from build123d import *

# Parameters (mm, degrees)
SKETCH1_R           = 2.0701
SKETCH1_R_2         = 2.4892
BOSS_EXTRUDE1_DEPTH = 2.54


with BuildPart() as part:
    # Sketch1 → Boss-Extrude1 (new body)
    with BuildSketch(Plane.XY):
        with BuildLine():
            Line((-35.539454624, 50.8), (60.96, 50.8))
            ThreePointArc((60.96, 50.8), (62.756051224, 50.056051224), (63.5, 48.26))
            Line((63.5, 48.26), (63.5, 27.94))
            ThreePointArc((63.5, 27.94), (62.756051224, 26.143948776), (60.96, 25.4))
            Line((60.96, 25.4), (39.37, 25.4))
            ThreePointArc((39.37, 25.4), (33.981846327, 23.168153673), (31.75, 17.78))
            Line((31.75, 17.78), (31.75, -3.81))
            ThreePointArc((31.75, -3.81), (31.006051224, -5.606051224), (29.21, -6.35))
            Line((29.21, -6.35), (-3.81, -6.35))
            ThreePointArc((-3.81, -6.35), (-5.606051224, -5.606051224), (-6.35, -3.81))
            Line((-6.35, -3.81), (-6.35, 17.78))
            ThreePointArc((-6.35, 17.78), (-8.581846327, 23.168153673), (-13.97, 25.4))
            Line((-13.97, 25.4), (-35.539454624, 25.4))
            ThreePointArc((-35.539454624, 25.4), (-37.335505848, 26.143948776), (-38.079454624, 27.94))
            Line((-38.079454624, 27.94), (-38.079454624, 48.26))
            ThreePointArc((-38.079454624, 48.26), (-37.335505848, 50.056051224), (-35.539454624, 50.8))
        make_face()
        with Locations((-25.4, 38.1)):
            Circle(SKETCH1_R, mode=Mode.SUBTRACT)
        with Locations((0, 38.1)):
            Circle(SKETCH1_R, mode=Mode.SUBTRACT)
        with Locations((25.4, 38.1)):
            Circle(SKETCH1_R, mode=Mode.SUBTRACT)
        with Locations((50.8, 38.1)):
            Circle(SKETCH1_R, mode=Mode.SUBTRACT)
        with Locations((0, 12.7)):
            Circle(SKETCH1_R_2, mode=Mode.SUBTRACT)
        Circle(SKETCH1_R_2, mode=Mode.SUBTRACT)
        with Locations((25.4, 12.7)):
            Circle(SKETCH1_R_2, mode=Mode.SUBTRACT)
        with Locations((25.4, 0)):
            Circle(SKETCH1_R_2, mode=Mode.SUBTRACT)
    extrude(amount=BOSS_EXTRUDE1_DEPTH)


solid = part.part
Input: part model. Units: mm. Frame: model coordinates. A direction names the side the tool comes from. Give positions to 0.01 mm unless a question says otherwise; leave off trailing zeros. Write each loop counter-clockwise with the first axis right and the second up, starting at its lowest first coordinate (ties: lowest second). Pieces come first, ordered by that corner, then holes. Notation, with made-up numbers: M 17,55 L 24,55 A13 cw 24,76 Z; hole C 77.5,78 d6. An arc over 180 degrees is marked long. Use one line per item in the form item = value.
1. Ray query, L1, parallel to Y at x = 0, z = 1.45; L2, parallel to X at y = 38.5, z = 0.5; L3, parallel to Y at x = -25.5, z = 0.3. Return the intervals inside material, ascending.
Outcome:
L1 = -6.35 to -2.49, 2.49 to 10.21, 15.19 to 36.03, 40.17 to 50.8
L2 = -38.08 to -27.43, -23.37 to -2.03, 2.03 to 23.37, 27.43 to 48.77, 52.83 to 63.5
L3 = 25.4 to 36.03, 40.17 to 50.8
2. Cut plane B-B on y = 38.1. Return loops of the section in (x, z), and give its area (3 significant figures).
Outcome:
outline = M -38.08,0 L -27.47,0 L -27.47,2.54 L -38.08,2.54 Z; M -23.33,0 L -2.07,0 L -2.07,2.54 L -23.33,2.54 Z; M 2.07,0 L 23.33,0 L 23.33,2.54 L 2.07,2.54 Z; M 27.47,0 L 48.73,0 L 48.73,2.54 L 27.47,2.54 Z; M 52.87,0 L 63.5,0 L 63.5,2.54 L 52.87,2.54 Z
area = 216 mm²
3. Cut plane D-D on z = 1.05. State how many separate pieces and enclosed holes the cut face has, and give its area (3 significant figures).
Outcome:
separate_pieces = 1
enclosed_holes = 8
area = 3,670 mm²
4. First-contact query: P1, Ø1.3, axis at x = 48, z = 1, coming from the -Y side; P2, Ø2.5, axis at x = 25.4, y = 38.1, coming from the +Z side; P3, Ø0.8, axis at y = 8, z = 1, coming from the +X side. Flat tips, straight axial feed; report the tip coordinate or a pass-through.
Outcome:
P1 = 25.4
P2 = through
P3 = 31.75
5. Mould query, pull axis Y, two halves, no side actions, for faces 4 (the face through (26.355, 36.263, 1.252)), 5 (the face through (-8.523, 23.109, 1.252)), 6 (the face through (-37.355, 50.036, 1.252)). Classes: released by +Y, released by -Y, zero draft, split by the parting line, or undercut.
Outcome:
face_4 = undercut
face_5 = released by -Y
face_6 = released by +Y
6. Cut plane A-A on x = -25.4. Return loops of the section in (y, z).
Outcome:
outline = M 25.4,0 L 36.03,0 L 36.03,2.54 L 25.4,2.54 Z; M 40.17,0 L 50.8,0 L 50.8,2.54 L 40.17,2.54 Z
7. Reachability of faces 1 (the face through (50, 25.4, 1)), 2 (the face through (-6.35, 7, 1)), 3 (the face through (63.5, 38, 1)) from +Z, -Z, +X, -X, +Y, -Y: full face, straight path, thin tool, end or side. Return the list, or none.
Outcome:
face_1 = +Z, -Z, +X, -Y
face_2 = +Z, -Z, -X, -Y
face_3 = +Z, -Z, +X, +Y, -Y
8. Cut plane C-C on x = 0. Return loops of the section in (y, z).
Outcome:
outline = M -6.35,0 L -2.49,0 L -2.49,2.54 L -6.35,2.54 Z; M 2.49,0 L 10.21,0 L 10.21,2.54 L 2.49,2.54 Z; M 15.19,0 L 36.03,0 L 36.03,2.54 L 15.19,2.54 Z; M 40.17,0 L 50.8,0 L 50.8,2.54 L 40.17,2.54 Z
